The listing builds one solid part. Answer for the finished solid, in the listing's coordinates (mm). Face numbers are marked on the shaded views. Coordinates: 2 decimals unless noted, no trailing zeros. Order: outer loops, then holes, each group sorted by start corner. A loop starts at its lowest first (then second) coordinate and runs counter-clockwise, first axis right, second up. Notation, with made-up numbers: (-35.5, 51.25) - (-24.5, 51.25) arc R18 cw to (-24.5, 81.25) - close; hole circle Ø2 at (-38.5, 1.5). An arc over 180 degrees is marked (long way). Use a Markdown table: item, result. Add a question column.
Item 1: Flat-ended cylindrical pins translate along their axes: P1, Ø0.6, axis at x = 0.5, z = 17.5, coming from the -Y side; P2, Ø6, axis at x = -27.5, z = 8, coming from the +Y side; P3, Ø3, axis at y = 15.5, z = 7.5, coming from the -X side. Find the tip coordinate at first contact, or state that the pin passes through.
Item 2: The part is cut by section C-C, the plane z = -6. Give the vertices of the cut face in (x, y), then the cut area to 3 significant figures.
Item 3: The part is cut by section A-A, the plane x = 44. Give the vertices of the cut face in (y, z) (3 decimals), then the cut area to 3 significant figures.
Item 4: The mould has two halves that part along X. Classify the marked faces 1, 2 and 3: released by +X, released by -X, zero draft, split by the parting line, or undercut.
Item 5: Find the intervals of material crossed by line 1 along X through (y, z) = (3.5, 15.5) (3 decimals); line 2 along Z through (x, y) = (-56.5, 10.5) (3 decimals); line 3 along X through (y, z) = (8, 9.5), in increasing order.
Item 6: The part is cut by section B-B, the plane z = 9. Give the vertices of the cut face in (x, y), then the cut area to 3 significant figures.
from build123d import *

# Parameters (mm, degrees)
SKETCH1_W            = 160.5788
SKETCH1_H            = 37.338
BOSS_EXTRUDE1_DEPTH  = 12.7
SKETCH2_W            = 157.5308
SKETCH2_H            = 34.29
CUT_EXTRUDE3_DEPTH   = 11.049
FILLET1_R            = 2.54
FILLET2_R            = 1.27
CUT_EXTRUDE4_REACH   = 164.158
SKETCH4_W            = 159.0548
SKETCH4_H            = 35.814
CUT_EXTRUDE5_DEPTH   = 1.778
FILLET3_R            = 1.524
SKETCH5_W            = 5.08
SKETCH5_H            = 0.762
BOSS_EXTRUDE2_DEPTH  = 7.62
SKETCH6_W            = 0.762
SKETCH6_H            = 2.032
BOSS_EXTRUDE3_DEPTH  = 13.589
LPATTERN1_COUNT      = 2
LPATTERN1_PITCH      = 101.6
LPATTERN1_COUNT_DIR2 = 2
LPATTERN1_PITCH_DIR2 = 32.258
CUT_EXTRUDE6_REACH   = 133.936
SKETCH8_W            = 3.81
SKETCH8_H            = 2.032
BOSS_EXTRUDE4_DEPTH  = 14.859
BOSS_EXTRUDE9_DEPTH  = 3.81
FILLET4_R            = 0.254
FILLET4_OF_MIRROR2_R = 0.254


with BuildPart() as part:
    # Sketch1 → Boss-Extrude1 (new body)
    with BuildSketch(Plane(origin=(0, 0, 0), x_dir=(1, 0, 0), z_dir=(0, 1, 0))):
        Rectangle(SKETCH1_W, SKETCH1_H)
    extrude(amount=BOSS_EXTRUDE1_DEPTH)

    # Sketch2 → Cut-Extrude3 (cut)
    with BuildSketch(Plane(origin=(0, 12.7, 0), x_dir=(1, 0, 0), z_dir=(0, 1, 0))):
        Rectangle(SKETCH2_W, SKETCH2_H)
    extrude(amount=-CUT_EXTRUDE3_DEPTH, mode=Mode.SUBTRACT)

    # Fillet1
    fillet1_edges = [part.edges().sort_by_distance(p)[0] for p in [
        (0, 0, 18.669),
        (-80.2894, 0, 0),
        (0, 0, -18.669),
        (80.2894, 0, 0),
        (80.2894, 6.35, 18.669),
        (-80.2894, 6.35, 18.669),
        (-80.2894, 6.35, -18.669),
        (80.2894, 6.35, -18.669),
    ]]
    fillet(fillet1_edges, radius=FILLET1_R)

    # Fillet2
    fillet2_edges = [part.edges().sort_by_distance(p)[0] for p in [
        (-78.7654, 7.1755, -17.145),
        (-78.7654, 7.1755, 17.145),
        (78.7654, 7.1755, 17.145),
        (78.7654, 7.1755, -17.145),
    ]]
    fillet(fillet2_edges, radius=FILLET2_R)

    # Sketch3 → Cut-Extrude4 (cut, up to next)
    with BuildSketch(Plane.ZY.offset(80.2894), mode=Mode.PRIVATE) as cut_extrude4_sk1:
        with BuildLine():
            Line((3.81, 3.8633146), (-3.81, 3.8633146))
            ThreePointArc((-3.81, 3.8633146), (-7.366, 7.4193146), (-3.81, 10.9753146))
            Line((-3.81, 10.9753146), (3.81, 10.9753146))
            ThreePointArc((3.81, 10.9753146), (7.366, 7.4193146), (3.81, 3.8633146))
        make_face()
    cut_extrude4_tool1 = extrude(cut_extrude4_sk1.sketch, amount=-CUT_EXTRUDE4_REACH, mode=Mode.PRIVATE) & part.part
    add(cut_extrude4_tool1.solids().sort_by_distance((-80.2894, 7.419315, 0))[0], mode=Mode.SUBTRACT)

    # Sketch4 → Cut-Extrude5 (cut)
    with BuildSketch(Plane(origin=(0, 12.7, 0), x_dir=(1, 0, 0), z_dir=(0, 1, 0))):
        Rectangle(SKETCH4_W, SKETCH4_H)
    extrude(amount=-CUT_EXTRUDE5_DEPTH, mode=Mode.SUBTRACT)

    # Fillet3
    fillet3_edges = [part.edges().sort_by_distance(p)[0] for p in [
        (-79.5274, 11.811, 17.907),
        (-79.5274, 11.811, -17.907),
        (79.5274, 11.811, -17.907),
        (79.5274, 11.811, 17.907),
    ]]
    fillet(fillet3_edges, radius=FILLET3_R)

    # Sketch5 → Boss-Extrude2 (add)
    with BuildSketch(Plane(origin=(0, 10.922, 0), x_dir=(1, 0, 0), z_dir=(0, 1, 0))):
        with Locations((-74.9554, -17.526)):
            Rectangle(SKETCH5_W, SKETCH5_H)
    extrude(amount=BOSS_EXTRUDE2_DEPTH)

    # Sketch6 → Boss-Extrude3 (add)
    with BuildSketch(Plane(origin=(0, 1.651, 0), x_dir=(1, 0, 0), z_dir=(0, 1, 0))):
        with Locations((-52.9844, 16.129)):
            Rectangle(SKETCH6_W, SKETCH6_H)
    boss_extrude3 = extrude(amount=BOSS_EXTRUDE3_DEPTH)

    # LPattern1: Boss-Extrude3 2 × 2
    with Locations(*[(i * LPATTERN1_PITCH, 0, j * LPATTERN1_PITCH_DIR2) for i in range(LPATTERN1_COUNT) for j in range(LPATTERN1_COUNT_DIR2) if (i, j) != (0, 0)]):
        add(boss_extrude3)

    # Cut-Extrude6: up to this face of the body (flat: up to its plane)
    cut_extrude6_end = Plane(part.part.faces().sort_by_distance((-53.3654, 8.4455, -16.129))[0])
    # Sketch7 → Cut-Extrude6 (cut, up to the picked face)
    with BuildSketch(Plane(origin=(48.9966, 0, 0), x_dir=(0, 0, -1), z_dir=(1, 0, 0)), mode=Mode.PRIVATE) as cut_extrude6_sk1:
        Polygon((17.145, 10.922), (15.494, 15.24), (17.145, 15.24), align=None)
    cut_extrude6_tool1 = split(extrude(cut_extrude6_sk1.sketch, amount=-CUT_EXTRUDE6_REACH, mode=Mode.PRIVATE), bisect_by=cut_extrude6_end, keep=Keep.BOTH, mode=Mode.PRIVATE)
    cut_extrude6 = cut_extrude6_tool1.solids().sort_by(Axis((48.9966, 13.800667, -16.594667), (-1, 0, 0)))[0]
    add(cut_extrude6, mode=Mode.SUBTRACT)

    # Mirror1: Cut-Extrude6 across plane
    add(cut_extrude6.mirror(Plane.XY), mode=Mode.SUBTRACT)

    # Sketch8 → Boss-Extrude4 (add)
    with BuildSketch(Plane(origin=(0, 1.651, 0), x_dir=(1, 0, 0), z_dir=(0, 1, 0))):
        with Locations((0, -16.129)):
            Rectangle(SKETCH8_W, SKETCH8_H)
        with Locations((0, 16.129)):
            Rectangle(SKETCH8_W, SKETCH8_H)
    extrude(amount=BOSS_EXTRUDE4_DEPTH)

    # Sketch9 → Boss-Extrude9 (add)
    with BuildSketch(Plane(origin=(1.905, 0, 0), x_dir=(0, 0, -1), z_dir=(1, 0, 0))):
        Polygon((-15.113, 16.51), (-17.907, 16.51), (-15.113, 18.542), align=None)
    boss_extrude9 = extrude(amount=-BOSS_EXTRUDE9_DEPTH)

    # Fillet4
    fillet4_edges = [part.edges().sort_by_distance(p)[0] for p in [
        (0, 18.542, 15.113),
    ]]
    fillet(fillet4_edges, radius=FILLET4_R)

    # Mirror2: Boss-Extrude9 across plane
    add(boss_extrude9.mirror(Plane.XY))

    # Fillet4 of Mirror2
    fillet4_of_mirror2_edges = [part.edges().sort_by_distance(p)[0] for p in [
        (0, 18.542, -15.113),
    ]]
    fillet(fillet4_of_mirror2_edges, radius=FILLET4_OF_MIRROR2_R)


solid = part.part
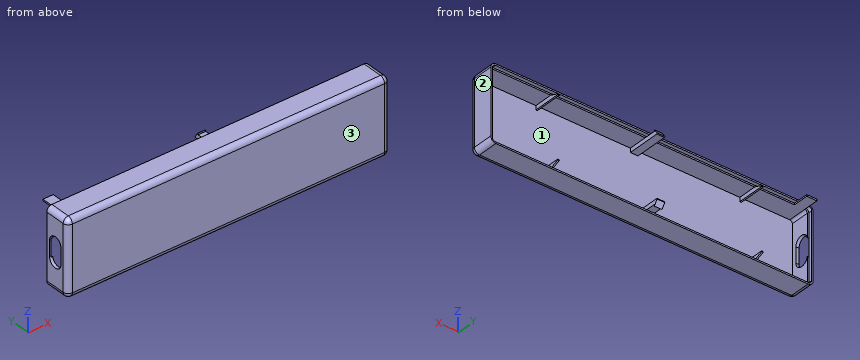
Solution:
| question | item | result |
|---|---|---|
| 1 | P1 | stops at y = 0.24 |
| 1 | P2 | stops at y = 1.65 |
| 1 | P3 | passes through |
| 2 | outline | (-80.29, 2.54) arc R2.54 ccw to (-77.75, 0) - (77.75, 0) arc R2.54 ccw to (80.29, 2.54) - (80.29, 12.7) - (79.53, 12.7) - (79.53, 10.92) - (78.77, 10.92) - (78.77, 1.65) - (-78.77, 1.65) - (-78.77, 4.62) - (-80.29, 4.62) - close; (-80.29, 10.22) - (-78.77, 10.22) - (-78.77, 10.92) - (-79.53, 10.92) - (-79.53, 12.7) - (-80.29, 12.7) - close |
| 2 | area | 285 mm2 |
| 3 | outline | (0, -16.129) arc R2.54 ccw to (2.54, -18.669) - (12.7, -18.669) - (12.7, -17.907) - (10.922, -17.907) - (10.922, -17.145) - (1.651, -17.145) - (1.651, 17.145) - (10.922, 17.145) - (10.922, 17.907) - (12.7, 17.907) - (12.7, 18.669) - (2.54, 18.669) arc R2.54 ccw to (0, 16.129) - close |
| 3 | area | 89.8 mm2 |
| 4 | face 1 | undercut |
| 4 | face 2 | released by +X |
| 4 | face 3 | zero draft |
| 5 | line 1 | x = -80.289 to -78.765, -53.365 to -52.603, -1.905 to 1.905, 48.235 to 48.997, 78.765 to 80.289 |
| 5 | line 2 | z = -18.669 to -17.145, 17.145 to 18.669 |
| 5 | line 3 | x = -80.29 to -78.77, 78.77 to 80.29 |
| 6 | outline | (-80.29, 2.54) arc R2.54 ccw to (-77.75, 0) - (77.75, 0) arc R2.54 ccw to (80.29, 2.54) - (80.29, 12.7) - (79.53, 12.7) - (79.53, 10.92) - (78.77, 10.92) - (78.77, 1.65) - (-78.77, 1.65) - (-78.77, 10.92) - (-79.53, 10.92) - (-79.53, 12.7) - (-80.29, 12.7) - close |
| 6 | area | 293 mm2 |
